```python
from build123d import *

# Parameters (mm, degrees)
SKETCH1_W                             = 87.3
SKETCH1_H                             = 93.65
BOSS_EXTRUDE1_DEPTH                   = 6.35
TAP_DRILL_FOR_M3X0_5_TAP1_D           = 2.5
TAP_DRILL_FOR_M3X0_5_TAP1_DEPTH       = 10
TAP_DRILL_FOR_M3X0_5_TAP1_CSINK_D     = 2.55
TAP_DRILL_FOR_M3X0_5_TAP1_CSINK_ANGLE = 90
TAP_DRILL_FOR_M3X0_5_TAP1_TIP         = 0.751075774
TAP_DRILL_FOR_M3X0_5_TAP2_D           = 2.5
TAP_DRILL_FOR_M3X0_5_TAP2_DEPTH       = 9.248924226
TAP_DRILL_FOR_M3X0_5_TAP2_CSINK_D     = 2.55
TAP_DRILL_FOR_M3X0_5_TAP2_CSINK_ANGLE = 90
TAP_DRILL_FOR_M3X0_5_TAP2_TIP         = 0.751075774
M3_CLEARANCE_HOLE2_D                  = 3.4
M3_CLEARANCE_HOLE2_CSINK_D            = 3.45
M3_CLEARANCE_HOLE2_CSINK_ANGLE        = 90


with BuildPart() as part:
    # Sketch1 → Boss-Extrude1 (new body)
    with BuildSketch(Plane(origin=(0, 0, 0), x_dir=(0, 0, -1), z_dir=(1, 0, 0))):
        Rectangle(SKETCH1_W, SKETCH1_H)
    extrude(amount=BOSS_EXTRUDE1_DEPTH)

    # Tap Drill for M3x0.5 Tap1
    with Locations(Plane(origin=(0, 46.825, 0), x_dir=(1, 0, 0), z_dir=(0, 1, 0))):
        with Locations((3.175, 35), (3.175, -35)):
            CounterSinkHole(TAP_DRILL_FOR_M3X0_5_TAP1_D / 2, TAP_DRILL_FOR_M3X0_5_TAP1_CSINK_D / 2, depth=TAP_DRILL_FOR_M3X0_5_TAP1_DEPTH, counter_sink_angle=TAP_DRILL_FOR_M3X0_5_TAP1_CSINK_ANGLE)
            with Locations((0, 0, -(TAP_DRILL_FOR_M3X0_5_TAP1_DEPTH + TAP_DRILL_FOR_M3X0_5_TAP1_TIP / 2))):  # 118° drill point
                Cone(0, TAP_DRILL_FOR_M3X0_5_TAP1_D / 2, TAP_DRILL_FOR_M3X0_5_TAP1_TIP, mode=Mode.SUBTRACT)

    # Tap Drill for M3x0.5 Tap2
    with Locations(Plane(origin=(0, -46.825, 0), x_dir=(-1, 0, 0), z_dir=(0, -1, 0))):
        with Locations((-3.175, -35), (-3.175, 35)):
            CounterSinkHole(TAP_DRILL_FOR_M3X0_5_TAP2_D / 2, TAP_DRILL_FOR_M3X0_5_TAP2_CSINK_D / 2, depth=TAP_DRILL_FOR_M3X0_5_TAP2_DEPTH, counter_sink_angle=TAP_DRILL_FOR_M3X0_5_TAP2_CSINK_ANGLE)
            with Locations((0, 0, -(TAP_DRILL_FOR_M3X0_5_TAP2_DEPTH + TAP_DRILL_FOR_M3X0_5_TAP2_TIP / 2))):  # 118° drill point
                Cone(0, TAP_DRILL_FOR_M3X0_5_TAP2_D / 2, TAP_DRILL_FOR_M3X0_5_TAP2_TIP, mode=Mode.SUBTRACT)

    # M3 Clearance Hole2 (through all)
    with Locations(Plane(origin=(6.35, 0, 0), x_dir=(0, 0, -1), z_dir=(1, 0, 0))):
        with Locations((-23.65, 36.825), (-10.48, 36.825), (-10.48, 8.885), (-23.65, 8.885)):
            CounterSinkHole(M3_CLEARANCE_HOLE2_D / 2, M3_CLEARANCE_HOLE2_CSINK_D / 2, counter_sink_angle=M3_CLEARANCE_HOLE2_CSINK_ANGLE)


solid = part.part
```
Could you check a few things on this model? Use its own coordinates, in mm. A direction names the side the tool comes from. Give positions to 0.01 mm unless a question says otherwise; leave off trailing zeros. Loops run counter-clockwise (first coordinate to the right, second up) from the corner with the lowest first, then second, coordinate; pieces in that order, holes last. Notation, with made-up numbers: (5, -13) - (33, -13) arc R19 cw to (33, 10) - close; hole circle Ø6 at (-7, 19). An arc over 180 degrees is marked (long way). Use one line per item in the form item = value.
1. I need wall thicknesses on probe 1 along Y at (x, z) = (3, 10.48) (3 decimals); probe 2 along X at (y, z) = (-43.5, -35) (3 decimals). Which ranges of each line are inside material? Lowest first, please.
Response values:
probe_1 = -46.825 to 7.185, 10.585 to 35.125, 38.525 to 46.825
probe_2 = 0 to 1.925, 4.425 to 6.35
2. I'm going to push flat-ended pins straight in: pin 1 Ø2 at (y, z) = (36.825, 10.48) entering from -X; pin 2 Ø1.5 at (x, z) = (3.175, -35) entering from -Y; pin 3 Ø2 at (x, z) = (3.175, 35) entering from -Y. Where does each tip first touch, or does it pass through?
Response values:
pin_1 = through
pin_2 = -37.28
pin_3 = -37.43
3. I want a section at A-A (z = 23.65). Please give me the cut outline in (x, y) (3 decimals).
Response values:
outline = (0, -46.825) - (6.35, -46.825) - (6.35, 7.16) - (6.325, 7.185) - (0, 7.185) - close; (0, 10.585) - (6.325, 10.585) - (6.35, 10.61) - (6.35, 35.1) - (6.325, 35.125) - (0, 35.125) - close; (0, 38.525) - (6.325, 38.525) - (6.35, 38.55) - (6.35, 46.825) - (0, 46.825) - close
4. Thinking about a two-plate mould opening in Y: for faces 4 (the face through (3.12, 36.17, 25.22)), 5 (the face through (3, 46.825, 1)), 6 (the face through (3.058, -36.955, 34.817)), which applies, released by +Y, released by -Y, zero draft, split by the parting line, or undercut?
Response values:
face_4 = undercut
face_5 = released by +Y
face_6 = released by -Y
5. On a 3-axis mill with a long thin cutter (end or side, diameter ignored), from which of +Z, -Z, +X, -X, +Y, -Y can I reach the whole of each face in a straight line? I mean faces 1 (the face through (3.45, 41.74, -33.78)), 2 (the face through (2.9, -42.12, -33.78)), 3 (the face through (3.1, 9.4, 12.1)). Say none if no direction works.
Response values:
face_1 = +Y
face_2 = -Y
face_3 = +X, -X
